Autodesk Inventor part; units mm, degrees
ref_plane "Work Plane1" through (20, 0, 0) normal (1, 0, 0) x (0, 1, 0)
ref_plane "XZ Plane" through (0, 0, 0) normal (0, 1, 0) x (-1, 0, 0)
ref_plane "XY Plane" through (0, 0, 0) normal (0, 0, 1) x (1, 0, 0)
sketch "Sketch1" plane through (0, 0, 0) normal (0, 1, 0) x (-1, 0, 0)
  circle A0 centre (0, 0) radius 20
  circle A1 centre (0, 0) radius 11.05
  dimension "d0" = 40
  dimension "d1" = 22.1
extrude "Extrusion1" add sketch "Sketch1" along normal blind 51.15
sketch "Sketch2" plane through (0, 0, 0) normal (0, -1, 0) x (1, 0, 0)
  circle A0 centre (0, 0) radius 13
  line L0 (0, 0) -> (9.1924, 0)
  line L1 (9.1924, 0) -> (9.1924, -9.1924)
  line L2 (9.1924, -9.1924) -> (0, -9.1924)
  line L3 (0, -9.1924) -> (0, 0)
  dimension "d4" = 26
  dimension "d5" = 9.1924
hole "Hole1" at (9.1924, 0, -9.1924) direction (0, 1, 0) diameter 2.2 depth 10 tip angle 118
pattern_circular "Circular Pattern1" count 4 over 360 about axis through (0, 0, 0) along (0, 1, 0) of "Hole1"
thread "Thread1"
thread "Thread3"
thread "Thread4"
thread "Thread5"
sketch "Sketch3" plane through (0, 51.15, 0) normal (0, 1, 0) x (1, 0, 0)
  circle A0 centre (0, 0) radius 20
  circle A1 centre (0, 0) radius 4.5
  dimension "d26" = 40
  dimension "d27" = 9
extrude "Extrusion2" add sketch "Sketch3" along normal blind 2
sketch "Sketch4" plane through (0, 53.15, 0) normal (0, 1, 0) x (1, 0, 0)
  point P0 (0, 0)
sketch "Sketch5" plane through (0, 53.15, 0) normal (0, 1, 0) x (1, 0, 0)
  circle A0 centre (0, 0) radius 6.75
  circle A1 centre (0, 0) radius 20
  dimension "d30" = 13.5
  dimension "d31" = 40
extrude "Extrusion3" add sketch "Sketch5" along normal blind 12
thread "Thread6"
sketch "Sketch8" plane through (0, 0, 0) normal (0, -1, 0) x (1, 0, 0)
  point P0 (0, 0)
sketch "Sketch9" plane through (0, 0, 0) normal (0, -1, 0) x (1, 0, 0)
  line L0 (0, 9.7277) -> (2.5, 9.7277)
  line L1 (2.5, 9.7277) -> (2.5, 16.3855)
  line L2 (2.5, 16.3855) -> (0, 16.3855)
  line L3 (0, 16.3855) -> (0, 9.7277)
  line L4 (0, 9.7277) -> (-2.5, 9.7277)
  line L5 (-2.5, 9.7277) -> (-2.5, 16.3855)
  line L6 (-2.5, 16.3855) -> (0, 16.3855)
  line L7 (0, 16.3855) -> (0, 9.7277)
  point P0 (0, 0)
  dimension "d1" = 22.1
  dimension "d54" = 2.5
  dimension "d55" = 2.5
extrude "Extrusion4" cut sketch "Sketch9" against normal blind 15
sketch "Sketch10" plane through (0, 0, 0) normal (1, 0, 0) x (0, 1, 0)
  point P0 (0, 0)
ref_plane "Work Plane1" through (20, 0, 0) normal (1, 0, 0) x (0, 1, 0)
sketch "Sketch15" plane through (0, 0, 0) normal (0, -1, 0) x (1, 0, 0)
  line L0 (2.5024, 10.6669) -> (-2.5, 10.6669)
  line L1 (-2.5, 10.6669) -> (-2.5, 24.5822)
  line L2 (-2.5, 24.5822) -> (2.5024, 24.5822)
  line L3 (2.5024, 24.5822) -> (2.5024, 10.6669)
  point P0 (0, 0)
extrude "Extrusion5" cut sketch "Sketch15" against normal blind 15
sketch "Sketch18" plane through (20, 0, 0) normal (1, 0, 0) x (0, 1, 0)
  line L0 (0, 0) -> (7.575, 0)
  line L1 (7.575, 0) -> (32.575, 0)
  line L2 (32.575, 0) -> (57.575, 0)
  dimension "d102" = 7.575
  dimension "d103" = 25
  dimension "d104" = 25
  dimension "d105" = 180
hole "Hole6" at (20, 57.575, 0) direction (-1, 0, 0) diameter 4 depth 8 tip angle 118
hole "Hole7" at (20, 7.575, 0) at (20, 32.575, 0) direction (-1, 0, 0) diameter 4 depth 8 tip angle 118
thread "Thread7"
thread "Thread8"
thread "Thread9"
sketch "Sketch19" plane through (0, 53.15, 0) normal (0, 1, 0) x (1, 0, 0)
  circle A0 centre (0, 0) radius 6.75
  circle A1 centre (0, 0) radius 6.4
  dimension "d128" = 13.5
  dimension "d129" = 12.8
extrude "Extrusion6" add sketch "Sketch19" along normal blind 2
thread "Thread11"
equation "\"d43\" = 60deg"
equation "\"Sketch6_Pitch\" = 0.5"
properties part number "enclosire2"
Source: CAD feature listing. Evaluate the final solid. Frame: model axes, mm. A direction names the side the tool comes from. Coordinates: 2 decimals unless noted, no trailing zeros. Write each loop counter-clockwise with the first axis right and the second up, starting at its lowest first coordinate (ties: lowest second). Pieces come first, ordered by that corner, then holes. Notation, with made-up numbers: M -16.5,65.25 L -11.5,65.25 A24 cw -11.5,79.25 Z; hole C -2,30 d7. An arc over 180 degrees is marked long. Use a Markdown table: item, result.
1) First-contact query: pin 1 Ø4 at (x, z) = (0, 16) entering from -Y; pin 2 Ø7.5 at (y, z) = (4, 17.5) entering from -X; pin 3 Ø15.5 at (x, z) = (0, 0) entering from -Y; pin 4 Ø6.5 at (y, z) = (32.575, 0) entering from +X. Flat tips, straight axial feed; report the tip coordinate or a pass-through.
Conclusion:
| item | result |
|---|---|
| pin 1 | stops at y = 15 |
| pin 2 | stops at x = -14.52 |
| pin 3 | stops at y = 51.15 |
| pin 4 | stops at x = 20 |
2) Reachability of faces 1 (the cylindrical face through (-0.59, 52.14, 4.46)), 2 (the cylindrical face through (15.94, 9.53, 0.43)), 3 (the cylindrical face through (10.21, 5.07, 9.61)) from +Z, -Z, +X, -X, +Y, -Y: full face, straight path, thin tool, end or side. Return the list, or none.
Conclusion:
| item | result |
|---|---|
| face 1 | +Y, -Y |
| face 2 | +X |
| face 3 | -Y |
3) Section A-A, the plane x = 0. Output: boundary loops of the cut face in (y, z).
Conclusion:
| item | result |
|---|---|
| outline | M 0,-20 L 65.15,-20 L 65.15,-6.75 L 55.15,-6.75 L 55.15,-6.4 L 53.15,-6.4 L 53.15,-4.5 L 51.15,-4.5 L 51.15,-11.05 L 0,-11.05 Z; M 15,11.05 L 51.15,11.05 L 51.15,4.5 L 53.15,4.5 L 53.15,6.4 L 55.15,6.4 L 55.15,6.75 L 65.15,6.75 L 65.15,20 L 15,20 Z |
4) Section C-C, the plane z = 3.5. Output: boundary loops of the cut face in (x, y), then the cut area to 3 significant figures.
Conclusion:
| item | result |
|---|---|
| outline | M -19.69,0 L -10.48,0 L -10.48,51.15 L -2.83,51.15 L -2.83,53.15 L -5.36,53.15 L -5.36,55.15 L -5.77,55.15 L -5.77,65.15 L -19.69,65.15 Z; M 2.83,51.15 L 10.48,51.15 L 10.48,0 L 19.69,0 L 19.69,65.15 L 5.77,65.15 L 5.77,55.15 L 5.36,55.15 L 5.36,53.15 L 2.83,53.15 Z |
| area | 1,350 mm^2 |
5) Mould query, pull axis X, two halves, no side actions, for faces 4 (the cylindrical face through (-5.94, 25.22, -9.32)), 5 (the flat face through (0, 0, -13)), 6 (the conical face through (11.01, 57.92, 0.05)), 7 (the cylindrical face through (-1.319, 32.119, -19.956)). Classes: pulls with the +X half, pulls with the -X half, needs draft (parallel to the pull), parting line crosses it, or undercut.
Conclusion:
| item | result |
|---|---|
| face 4 | undercut |
| face 5 | needs draft |
| face 6 | pulls with the +X half |
| face 7 | parting line crosses it |
6) Ray query, L1, parallel to Y at x = 15, z = 0 (3 decimals); L2, parallel to Z at x = 0, y = 54.1. Return the intervals inside material, ascending.
Conclusion:
| item | result |
|---|---|
| L1 | y = 0 to 5.575, 9.575 to 30.575, 34.575 to 55.575, 59.575 to 65.15 |
| L2 | z = -20 to -6.4, 6.4 to 20 |
7) Section B-B, the plane z = 16. Output: boundary loops of the cut face in (x, y).
Conclusion:
| item | result |
|---|---|
| outline | M -12,0 L -2.5,0 L -2.5,15 L 2.5,15 L 2.5,0 L 12,0 L 12,65.15 L -12,65.15 Z |
8) Section D-D, the plane x = 15.5. Output: boundary loops of the cut face in (y, z) (3 decimals), then the cut area to 3 significant figures.
Conclusion:
| item | result |
|---|---|
| outline | M 0,-12.639 L 65.15,-12.639 L 65.15,12.639 L 0,12.639 Z; hole C 7.575,0 d4; hole C 32.575,0 d4; hole C 57.575,0 d4 |
| area | 1,610 mm^2 |
